Design review of the part built by this model. Coordinates are the model's own, in mm. Face numbers are marked on the shaded views. A direction names the side the tool comes from. Coordinates: 2 decimals unless noted, no trailing zeros. Write each loop counter-clockwise with the first axis right and the second up, starting at its lowest first coordinate (ties: lowest second). Pieces come first, ordered by that corner, then holes. Notation, with made-up numbers: M 20.25,39 L 61.25,39 A13 cw 61.25,60 Z; hole C -32,19.5 d3. An arc over 180 degrees is marked long. Return JSON: item names as keys, results as strings. Group by question number.
```python
from build123d import *

# Parameters (mm, degrees)
F2_R     = 140
F2_R_2   = 11.1
F2_R_3   = 107.95
F4_DEPTH = 23.9
F5_DEPTH = 25.5


# Not quite as in the source:
# - a feature names something its author has since deleted; it is built from what else it names


with BuildPart() as f4:
    # F2 (on Top) → F4 (new body)
    with BuildSketch(Plane.XY):
        Circle(F2_R)
        with Locations((-46.1707561148, -111.4660655975)):
            Circle(F2_R_2, mode=Mode.SUBTRACT)
        with Locations((-111.4660655975, -46.1707561148)):
            Circle(F2_R_2, mode=Mode.SUBTRACT)
        with Locations((46.1707561148, -111.4660655975)):
            Circle(F2_R_2, mode=Mode.SUBTRACT)
        with Locations((111.4660655975, -46.1707561148)):
            Circle(F2_R_2, mode=Mode.SUBTRACT)
        with Locations((-111.4660655975, 46.1707561148)):
            Circle(F2_R_2, mode=Mode.SUBTRACT)
        with Locations((-46.1707561148, 111.4660655975)):
            Circle(F2_R_2, mode=Mode.SUBTRACT)
        Circle(F2_R_3, mode=Mode.SUBTRACT)
        with Locations((111.4660655975, 46.1707561148)):
            Circle(F2_R_2, mode=Mode.SUBTRACT)
        with Locations((46.1707561148, 111.4660655975)):
            Circle(F2_R_2, mode=Mode.SUBTRACT)
        Circle(F2_R_3)
    extrude(amount=F4_DEPTH)

    # F2 (on Top) → F5 (join)
    with BuildSketch(Plane.XY):
        Circle(F2_R_3)
    extrude(amount=F5_DEPTH)


solid = f4.part
```
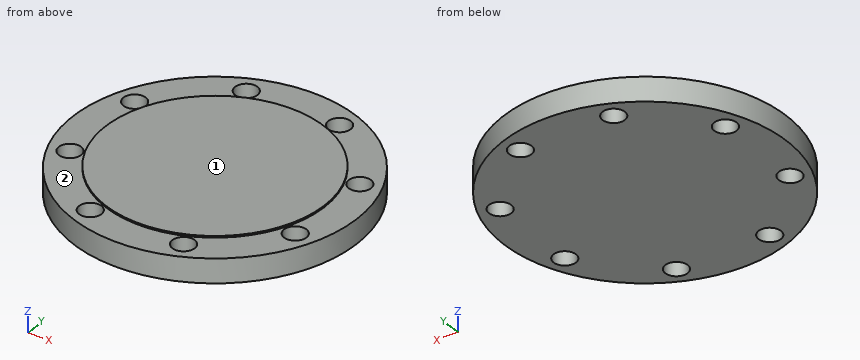
Item 1: Add section A-A (y = 91.5). Write out the cut boundary in (x, z), plus the area to 3 significant figures.
Item 2: Add section C-C (x = -14.5). Write out the cut boundary in (y, z).
Item 3: For pin 1 (3 mm diameter, centred on x = 99.5, y = -45, fed in from +Z); pin 2 (3 mm diameter, centred on y = -104.5, z = 4, fed in from -X); pin 3 (2 mm diameter, centred on x = 55.5, z = 4.5, fed in from -Y); pin 4 (8 mm diameter, centred on x = -36.5, z = 9.5, fed in from +Y), all flat-tipped, find the tip position at first contact; note any pin that passes through.
Item 4: Machinability: for the marked faces 1 and 2, which of the approach directions +Z, -Z, +X, -X, +Y, -Y give a long, thin tool a straight path to every point of the face, cutting with its end or side? Answer none if there is none.
Item 5: Add section B-B (z = 8.5). Count the separate pieces of the cut face and the enclosed holes in it, plus the area to 3 significant figures.
Item 6: For line 1 (Y direction, x = 106, z = 23.5); line 2 (X direction, y = 49.5, z = 13.5); line 3 (Y direction, x = 114.5, z = 16.5), list the stretches that pass through material, from the lowest coordinate up.
Geometry check:
{
 "1": {"outline": "M -105.96,0 L 105.96,0 L 105.96,23.9 L 57.28,23.9 L 57.28,25.5 L -57.28,25.5 L -57.28,23.9 L -105.96,23.9 Z", "area": "5,250 mm^2"},
 "2": {"outline": "M -139.25,0 L 139.25,0 L 139.25,23.9 L 106.97,23.9 L 106.97,25.5 L -106.97,25.5 L -106.97,23.9 L -139.25,23.9 Z"},
 "3": {"pin 1": "z = 25.5", "pin 2": "x = -94.82", "pin 3": "y = -128.96", "pin 4": "y = 136.18"},
 "4": {"face 1": "+Z, +X, -X, +Y, -Y", "face 2": "+Z"},
 "5": {"separate pieces": "1", "enclosed holes": "8", "area": "58,500 mm^2"},
 "6": {"line 1": "-91.45 to -55.83, -36.51 to 36.51, 55.83 to 91.45", "line 2": "-130.96 to -122.06, -100.88 to 100.88, 122.06 to 130.96", "line 3": "-80.56 to -56.85, -35.49 to 35.49, 56.85 to 80.56"}
}
